from build123d import *

# Parameters (mm, degrees)
F0_W     = 1270
F0_H     = 19.05
F0_W_2   = 1.905
F0_H_2   = 482.6
F0_H_3   = 152.4
F0_H_4   = 812.8
F0_W_3   = 381.635
F1_DEPTH = 812.8
F3_START = -812.8
F2_W     = 1308.1
F2_H     = 2216.15
F3_DEPTH = 1.905


# Not quite as in the source:
# - a feature names something its author has since deleted; it is built from what else it names


with BuildPart() as f1:
    # F0 (on Front) → F1 (new body)
    with BuildSketch(Plane.XZ):
        Polygon((-635, -396.875), (-635, 415.925), (-635, 434.975), (-635, 841.375), (-635, 860.425), (-635, 1012.825), (-635, 1031.875), (-635, 1108.075), (-635, 1127.125), (-635, 1279.525), (-635, 1298.575), (-654.05, 1298.575), (-654.05, -917.575), (-635, -917.575), (-635, -898.525), (-635, -415.925), align=None)
        Polygon((-635, 434.975), (-635, 415.925), (404.495, 415.925), (406.4, 415.925), (635, 415.925), (635, 434.975), align=None)
        Polygon((-635, 860.425), (-635, 841.375), (635, 841.375), (635, 860.425), (332.105, 860.425), (330.2, 860.425), (0, 860.425), align=None)
        Polygon((-635, 1031.875), (-635, 1012.825), (0, 1012.825), (330.2, 1012.825), (332.105, 1012.825), (635, 1012.825), (635, 1031.875), align=None)
        with Locations((0, 1289.05)):
            Rectangle(F0_W, F0_H)
        Polygon((635, 841.375), (635, 434.975), (635, 415.925), (635, -396.875), (635, -415.925), (635, -647.7), (635, -666.75), (635, -898.525), (635, -917.575), (654.05, -917.575), (654.05, 1298.575), (635, 1298.575), (635, 1279.525), (635, 1127.125), (635, 1108.075), (635, 1031.875), (635, 1012.825), (635, 860.425), align=None)
        Polygon((404.495, -396.875), (-635, -396.875), (-635, -415.925), (-431.8, -415.925), (-429.895, -415.925), (-226.695, -415.925), (-224.79, -415.925), (-21.59, -415.925), (-19.685, -415.925), (234.315, -415.925), (253.365, -415.925), (635, -415.925), (635, -396.875), (406.4, -396.875), align=None)
        Polygon((-431.8, -898.525), (-635, -898.525), (-635, -917.575), (635, -917.575), (635, -898.525), (253.365, -898.525), (234.315, -898.525), (-19.685, -898.525), (-21.59, -898.525), (-224.79, -898.525), (-226.695, -898.525), (-429.895, -898.525), align=None)
        with Locations((-430.8475, -657.225)):
            Rectangle(F0_W_2, F0_H_2)
        with Locations((-225.7425, -657.225)):
            Rectangle(F0_W_2, F0_H_2)
        with Locations((-20.6375, -657.225)):
            Rectangle(F0_W_2, F0_H_2)
        with Locations((0, 1117.6)):
            Rectangle(F0_W, F0_H)
        with Locations((331.1525, 936.625)):
            Rectangle(F0_W_2, F0_H_3)
        with Locations((405.4475, 9.525)):
            Rectangle(F0_W_2, F0_H_4)
        Polygon((253.365, -647.7), (253.365, -415.925), (234.315, -415.925), (234.315, -898.525), (253.365, -898.525), (253.365, -666.75), align=None)
        with Locations((444.1825, -657.225)):
            Rectangle(F0_W_3, F0_H)
    extrude(amount=F1_DEPTH)

    # F2 (on face) → F3 (join)
    with BuildSketch(Plane.XZ.offset(812.8).offset(F3_START)):
        with Locations((0, 190.5)):
            Rectangle(F2_W, F2_H)
    extrude(amount=-F3_DEPTH)


solid = f1.part
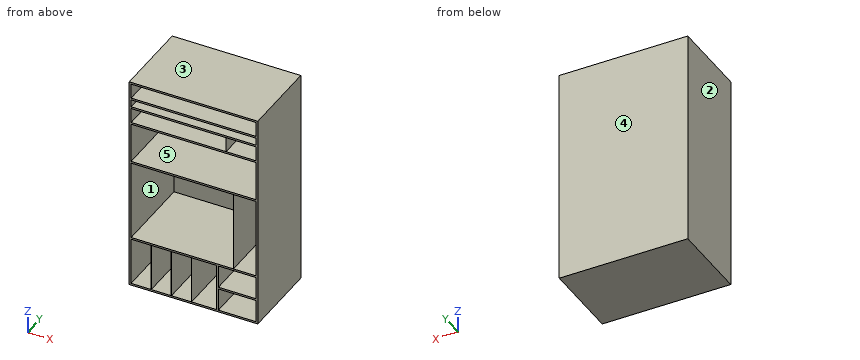
Model file for the job. Use its own axes, mm. Face numbers are marked on the shaded views. A direction names the side the tool comes from. Give positions to 0.01 mm unless a question says otherwise; leave off trailing zeros. Loops run counter-clockwise (first coordinate to the right, second up) from the corner with the lowest first, then second, coordinate; pieces in that order, holes last. Notation, with made-up numbers: (-18, 10.25) - (1, 10.25) arc R16 cw to (1, 35.25) - close; hole circle Ø11 at (11.5, 29). An arc over 180 degrees is marked (long way). Use one line per item in the form item = value.
(1) Drill centre lines: L1, parallel to X at y = -95, z = 286 (3 decimals); L2, parallel to X at y = -761, z = -703.5 (3 decimals); L3, parallel to X at y = -375, z = 893 (3 decimals). Where is each one in solid material? Low to high.
Determined:
L1 = -654.05 to -635, 404.495 to 406.4, 635 to 654.05
L2 = -654.05 to -635, -431.8 to -429.895, -226.695 to -224.79, -21.59 to -19.685, 234.315 to 253.365, 635 to 654.05
L3 = -654.05 to -635, 330.2 to 332.105, 635 to 654.05
(2) Cut at C-C (y = -432.5). Count the separate pieces of the cut face and the enclosed holes in it, then the cut area to 3 significant figures.
Determined:
separate_pieces = 1
enclosed_holes = 13
area = 275,000 mm^2
(3) Cut at A-A (z = 347). Give the cut face in (x, y) (3 decimals).
Determined:
outline = (-654.05, -812.8) - (-635, -812.8) - (-635, 0) - (404.495, 0) - (404.495, -812.8) - (406.4, -812.8) - (406.4, 0) - (635, 0) - (635, -812.8) - (654.05, -812.8) - (654.05, 1.905) - (-654.05, 1.905) - close
(4) Pull direction X, two halves, no side cores. Call the marked faces 1, 2 and 3: pulls with the +X half, pulls with the -X half, needs draft (parallel to the pull), parting line crosses it, or undercut.
Determined:
face_1 = undercut
face_2 = pulls with the -X half
face_3 = needs draft
(5) 3-axis set-ups, long thin cutter, end or side, ignore diameter. For the marked faces 4 and 5: which of +Z, -Z, +X, -X, +Y, -Y reach the whole face in a straight line?
Determined:
face_4 = +Z, -Z, +X, -X, +Y
face_5 = -Y
(6) Cut at D-D (z = -710). Give the cut face in (x, y) (3 decimals), then the cut area to 3 significant figures.
Determined:
outline = (-654.05, -812.8) - (-635, -812.8) - (-635, 0) - (-431.8, 0) - (-431.8, -812.8) - (-429.895, -812.8) - (-429.895, 0) - (-226.695, 0) - (-226.695, -812.8) - (-224.79, -812.8) - (-224.79, 0) - (-21.59, 0) - (-21.59, -812.8) - (-19.685, -812.8) - (-19.685, 0) - (234.315, 0) - (234.315, -812.8) - (253.365, -812.8) - (253.365, 0) - (635, 0) - (635, -812.8) - (654.05, -812.8) - (654.05, 1.905) - (-654.05, 1.905) - close
area = 53,600 mm^2
(7) Drop a flat-ended pin along its axis: P1, Ø4, axis at x = 87, z = -548, coming from the -Y side. Give the stop position or say it passes through.
Determined:
P1 = 0
(8) Cut at B-B (x = -475). Give the cut face in (y, z) (3 decimals).
Determined:
outline = (-812.8, -917.575) - (1.905, -917.575) - (1.905, 1298.575) - (-812.8, 1298.575) - (-812.8, 1279.525) - (0, 1279.525) - (0, 1127.125) - (-812.8, 1127.125) - (-812.8, 1108.075) - (0, 1108.075) - (0, 1031.875) - (-812.8, 1031.875) - (-812.8, 1012.825) - (0, 1012.825) - (0, 860.425) - (-812.8, 860.425) - (-812.8, 841.375) - (0, 841.375) - (0, 434.975) - (-812.8, 434.975) - (-812.8, 415.925) - (0, 415.925) - (0, -396.875) - (-812.8, -396.875) - (-812.8, -415.925) - (0, -415.925) - (0, -898.525) - (-812.8, -898.525) - close
